from build123d import *

# Parameters (mm, degrees)
SALIENTE_EXTRUIR1_DEPTH    = 4
CROQUIS2_W                 = 55
CROQUIS2_H                 = 61
CORTAR_EXTRUIR1_DEPTH      = 2
CROQUIS12_W                = 3
CROQUIS12_H                = 11
SALIENTE_EXTRUIR2_DEPTH    = 15
CROQUIS13_W                = 5
CROQUIS13_H                = 12
CORTAR_EXTRUIR8_DEPTH      = 80
CORTAR_EXTRUIR8_DEPTH_BACK = 4
CROQUIS14_W                = 5
CROQUIS14_H                = 12
CORTAR_EXTRUIR9_DEPTH      = 80
CORTAR_EXTRUIR9_DEPTH_BACK = 4
CROQUIS15_W                = 35
CROQUIS15_H                = 10
CORTAR_EXTRUIR10_DEPTH     = 20


with BuildPart() as part:
    # Croquis1 → Saliente-Extruir1 (new body)
    with BuildSketch(Plane(origin=(0, 0, 0), x_dir=(1, 0, 0), z_dir=(0, 1, 0))):
        Polygon((30, -32.5), (30, -22.5), (41, -22.5), (41, -11.5), (30, -11.5), (30, 11.5), (41, 11.5), (41, 22.5), (30, 22.5), (30, 32.5), (-30, 32.5), (-30, 22.5), (-41, 22.5), (-41, 11.5), (-30, 11.5), (-30, -11.5), (-41, -11.5), (-41, -22.5), (-30, -22.5), (-30, -32.5), align=None)
    extrude(amount=SALIENTE_EXTRUIR1_DEPTH)

    # Croquis2 → Cortar-Extruir1 (cut)
    with BuildSketch(Plane(origin=(0, 4, 0), x_dir=(1, 0, 0), z_dir=(0, 1, 0))):
        Rectangle(CROQUIS2_W, CROQUIS2_H)
    extrude(amount=-CORTAR_EXTRUIR1_DEPTH, mode=Mode.SUBTRACT)

    # Croquis12 → Saliente-Extruir2 (add)
    with BuildSketch(Plane(origin=(0, 4, 0), x_dir=(1, 0, 0), z_dir=(0, 1, 0))):
        with Locations((-39.5, 17)):
            Rectangle(CROQUIS12_W, CROQUIS12_H)
        with Locations((-39.5, -17)):
            Rectangle(CROQUIS12_W, CROQUIS12_H)
        with Locations((39.5, -17)):
            Rectangle(CROQUIS12_W, CROQUIS12_H)
        with Locations((39.5, 17)):
            Rectangle(CROQUIS12_W, CROQUIS12_H)
    extrude(amount=SALIENTE_EXTRUIR2_DEPTH)

    # Croquis13 → Cortar-Extruir8 (cut, two sides)
    with BuildSketch(Plane.ZY.offset(-38)) as cortar_extruir8_sk:
        with Locations((-17, 10)):
            Rectangle(CROQUIS13_W, CROQUIS13_H)
    extrude(amount=CORTAR_EXTRUIR8_DEPTH, mode=Mode.SUBTRACT)
    extrude(cortar_extruir8_sk.sketch, amount=-CORTAR_EXTRUIR8_DEPTH_BACK, mode=Mode.SUBTRACT)

    # Croquis14 → Cortar-Extruir9 (cut, two sides)
    with BuildSketch(Plane.ZY.offset(-38)) as cortar_extruir9_sk:
        with Locations((17, 10)):
            Rectangle(CROQUIS14_W, CROQUIS14_H)
    extrude(amount=CORTAR_EXTRUIR9_DEPTH, mode=Mode.SUBTRACT)
    extrude(cortar_extruir9_sk.sketch, amount=-CORTAR_EXTRUIR9_DEPTH_BACK, mode=Mode.SUBTRACT)

    # Croquis15 → Cortar-Extruir10 (cut, through all)
    with BuildSketch(Plane(origin=(0, 0, 0), x_dir=(1, 0, 0), z_dir=(0, 1, 0))):
        Rectangle(CROQUIS15_W, CROQUIS15_H)
        with Locations((0, -18)):
            Rectangle(CROQUIS15_W, CROQUIS15_H)
        with Locations((0, 18)):
            Rectangle(CROQUIS15_W, CROQUIS15_H)
    extrude(amount=CORTAR_EXTRUIR10_DEPTH, mode=Mode.SUBTRACT)


solid = part.part
Verification items for the finished model (mm, model axes). A direction names the side the tool comes from. Round coordinates to 2 decimals unless told otherwise and drop trailing zeros. Write each loop counter-clockwise with the first axis right and the second up, starting at its lowest first coordinate (ties: lowest second). Pieces come first, ordered by that corner, then holes.
(1) Section check A-A (y = 10.5). Give the number of separate pieces and of enclosed holes in the cut face, plus the area to 3 significant figures.
Returned:
separate pieces: 8
enclosed holes: 0
area: 72.0 mm2
(2) Access from +Z, -Z, +X, -X, +Y, -Y to the whole of each face (thin tool, end or side, straight path). Record for faces 4 (the flat face through (-39, 16, -17)), 5 (the flat face through (-17.5, 1, 18)), 6 (the flat face through (0, 2, -7)).
Returned:
face 4: +X, -X
face 5: +Y, -Y
face 6: +Y
(3) Material ranges on line 1 (Z direction, x = 23, y = 3.25); line 2 (Z direction, x = -10.5, y = 1.5); line 3 (X direction, y = 1, z = -20), recorded low to high.
Returned:
line 1: z = -32.5 to -30.5, 30.5 to 32.5
line 2: z = -32.5 to -23, -13 to -5, 5 to 13, 23 to 32.5
line 3: x = -41 to -17.5, 17.5 to 41
(4) Depth check by flat-ended pin: pin 1 Ø1.5 at (x, z) = (-18, 9) entering from +Y; pin 2 Ø2 at (y, z) = (2.5, -29.5) entering from -X; pin 3 Ø3 at (x, z) = (29.5, 23) entering from +Y. Enter the tip coordinate at first touch or a pass-through.
Returned:
pin 1: stops at y = 2
pin 2: stops at x = -30
pin 3: stops at y = 4
(5) Mould release check, pull along Z, two halves, no side actions. Record for faces 1 (the flat face through (39, 5, 22.5)), 2 (the flat face through (-39, 7, -11.5)), 3 (the flat face through (-30, 2, 27)): pulls with the +Z half, pulls with the -Z half, needs draft (parallel to the pull), parting line crosses it, or undercut.
Returned:
face 1: pulls with the +Z half
face 2: undercut
face 3: needs draft
(6) Section check B-B (x = -7). Enter the section's corners in (y, z).
Returned:
outline: (0, -32.5) - (4, -32.5) - (4, -30.5) - (2, -30.5) - (2, -23) - (0, -23) - close; (0, -13) - (2, -13) - (2, -5) - (0, -5) - close; (0, 5) - (2, 5) - (2, 13) - (0, 13) - close; (0, 23) - (2, 23) - (2, 30.5) - (4, 30.5) - (4, 32.5) - (0, 32.5) - close
(7) Section check D-D (y = 3). Enter the section's corners in (x, z).
Returned:
outline: (-41, -22.5) - (-30, -22.5) - (-30, -32.5) - (30, -32.5) - (30, -22.5) - (41, -22.5) - (41, -11.5) - (30, -11.5) - (30, 11.5) - (41, 11.5) - (41, 22.5) - (30, 22.5) - (30, 32.5) - (-30, 32.5) - (-30, 22.5) - (-41, 22.5) - (-41, 11.5) - (-30, 11.5) - (-30, -11.5) - (-41, -11.5) - close; hole (-27.5, -30.5) - (27.5, -30.5) - (27.5, 30.5) - (-27.5, 30.5) - close
(8) Section check C-C (z = -15.5). Enter the section's corners in (x, y).
Returned:
outline: (-41, 0) - (-17.5, 0) - (-17.5, 2) - (-27.5, 2) - (-27.5, 4) - (-41, 4) - close; (-41, 16) - (-38, 16) - (-38, 19) - (-41, 19) - close; (17.5, 0) - (41, 0) - (41, 4) - (27.5, 4) - (27.5, 2) - (17.5, 2) - close; (38, 16) - (41, 16) - (41, 19) - (38, 19) - close
